Check sheet for the modelled part. Datum: model origin and axes. Units: mm. Give positions to 0.01 mm unless a question says otherwise; leave off trailing zeros. Order: outer loops, then holes, each group sorted by start corner. A loop starts at its lowest first (then second) coordinate and runs counter-clockwise, first axis right, second up.
Item 1: Material ranges on line 1 along X through (y, z) = (40, 1.9); line 2 along Y through (x, z) = (-79.5, 2.5); line 3 along X through (y, z) = (-140, 2.8), recorded low to high.
Item 2: Sectioned sample at C-C on z = 2. Count the separate pieces of the cut face and the enclosed holes in it, and give its area (3 significant figures).
Item 3: Sectioned sample at A-A on x = 3. Record the boundary of the cut face in (y, z) (3 decimals), and give its area (3 significant figures).
Item 4: Sectioned sample at B-B on x = 147. Record the boundary of the cut face in (y, z) (3 decimals).
from build123d import *

# Parameters (mm, degrees)
F0_R     = 1.984375
F0_W     = 38.1
F0_H     = 3.302
F0_W_2   = 3.302
F0_H_2   = 50.8
F0_W_3   = 79.248
F0_H_3   = 275.232702
F0_W_4   = 152.4
F0_H_4   = 254
F1_DEPTH = 3.175


with BuildPart() as f1:
    # F0 (on Top) → F1 (new body)
    with BuildSketch(Plane.XY):
        Polygon((-107.700216, 150.306364), (-206.125216, 150.306364), (-206.125216, -167.193636), (-107.700216, -167.193636), (114.549784, -167.193636), (212.974784, -167.193636), (212.974784, 150.306364), (114.549784, 150.306364), align=None)
        with Locations((-199.775216, -110.043636)):
            Circle(F0_R, mode=Mode.SUBTRACT)
        with Locations((-199.775216, -97.343636)):
            Circle(F0_R, mode=Mode.SUBTRACT)
        with Locations((-85.475216, -151.191636)):
            Circle(F0_R, mode=Mode.SUBTRACT)
        with Locations((-66.171216, -159.192636)):
            Rectangle(F0_W, F0_H, mode=Mode.SUBTRACT)
        with Locations((-72.775216, -151.191636)):
            Circle(F0_R, mode=Mode.SUBTRACT)
        with Locations((-60.075216, -151.191636)):
            Circle(F0_R, mode=Mode.SUBTRACT)
        with Locations((-47.375216, -151.191636)):
            Circle(F0_R, mode=Mode.SUBTRACT)
        with Locations((-34.675216, -151.191636)):
            Circle(F0_R, mode=Mode.SUBTRACT)
        with Locations((3.424784, -159.192636)):
            Rectangle(F0_W, F0_H, mode=Mode.SUBTRACT)
        with Locations((-199.775216, -84.643636)):
            Circle(F0_R, mode=Mode.SUBTRACT)
        with Locations((-191.774216, -84.643636)):
            Rectangle(F0_W_2, F0_H_2, mode=Mode.SUBTRACT)
        with Locations((-199.775216, -71.943636)):
            Circle(F0_R, mode=Mode.SUBTRACT)
        with Locations((-199.775216, -59.243636)):
            Circle(F0_R, mode=Mode.SUBTRACT)
        with Locations((-102.874216, -84.643636)):
            Rectangle(F0_W_2, F0_H_2, mode=Mode.SUBTRACT)
        with Locations((-86.872216, -84.643636)):
            Rectangle(F0_W_2, F0_H_2, mode=Mode.SUBTRACT)
        with Locations((41.524784, -151.191636)):
            Circle(F0_R, mode=Mode.SUBTRACT)
        with Locations((54.224784, -151.191636)):
            Circle(F0_R, mode=Mode.SUBTRACT)
        with Locations((73.020784, -159.192636)):
            Rectangle(F0_W, F0_H, mode=Mode.SUBTRACT)
        with Locations((66.924784, -151.191636)):
            Circle(F0_R, mode=Mode.SUBTRACT)
        with Locations((79.624784, -151.191636)):
            Circle(F0_R, mode=Mode.SUBTRACT)
        with Locations((92.324784, -151.191636)):
            Circle(F0_R, mode=Mode.SUBTRACT)
        with Locations((206.624784, -110.043636)):
            Circle(F0_R, mode=Mode.SUBTRACT)
        with Locations((206.624784, -97.343636)):
            Circle(F0_R, mode=Mode.SUBTRACT)
        with Locations((93.721784, -84.643636)):
            Rectangle(F0_W_2, F0_H_2, mode=Mode.SUBTRACT)
        with Locations((109.723784, -84.643636)):
            Rectangle(F0_W_2, F0_H_2, mode=Mode.SUBTRACT)
        with Locations((198.623784, -84.643636)):
            Rectangle(F0_W_2, F0_H_2, mode=Mode.SUBTRACT)
        with Locations((206.624784, -84.643636)):
            Circle(F0_R, mode=Mode.SUBTRACT)
        with Locations((206.624784, -71.943636)):
            Circle(F0_R, mode=Mode.SUBTRACT)
        with Locations((206.624784, -59.243636)):
            Circle(F0_R, mode=Mode.SUBTRACT)
        with Locations((-191.774216, -8.443636)):
            Rectangle(F0_W_2, F0_H_2, mode=Mode.SUBTRACT)
        with Locations((-147.324216, -5.242554)):
            Rectangle(F0_W_3, F0_H_3, mode=Mode.SUBTRACT)
        with Locations((-102.874216, -8.443636)):
            Rectangle(F0_W_2, F0_H_2, mode=Mode.SUBTRACT)
        with Locations((-199.775216, 42.356364)):
            Circle(F0_R, mode=Mode.SUBTRACT)
        with Locations((-199.775216, 55.056364)):
            Circle(F0_R, mode=Mode.SUBTRACT)
        with Locations((-199.775216, 67.756364)):
            Circle(F0_R, mode=Mode.SUBTRACT)
        with Locations((-191.774216, 67.756364)):
            Rectangle(F0_W_2, F0_H_2, mode=Mode.SUBTRACT)
        with Locations((-102.874216, 67.756364)):
            Rectangle(F0_W_2, F0_H_2, mode=Mode.SUBTRACT)
        with Locations((-86.872216, -8.443636)):
            Rectangle(F0_W_2, F0_H_2, mode=Mode.SUBTRACT)
        with Locations((3.424784, -8.443636)):
            Rectangle(F0_W_4, F0_H_4, mode=Mode.SUBTRACT)
        with Locations((-86.872216, 67.756364)):
            Rectangle(F0_W_2, F0_H_2, mode=Mode.SUBTRACT)
        with Locations((-199.775216, 80.456364)):
            Circle(F0_R, mode=Mode.SUBTRACT)
        with Locations((-199.775216, 93.156364)):
            Circle(F0_R, mode=Mode.SUBTRACT)
        with Locations((-85.475216, 134.304364)):
            Circle(F0_R, mode=Mode.SUBTRACT)
        with Locations((-72.775216, 134.304364)):
            Circle(F0_R, mode=Mode.SUBTRACT)
        with Locations((-60.075216, 134.304364)):
            Circle(F0_R, mode=Mode.SUBTRACT)
        with Locations((-66.171216, 142.305364)):
            Rectangle(F0_W, F0_H, mode=Mode.SUBTRACT)
        with Locations((-47.375216, 134.304364)):
            Circle(F0_R, mode=Mode.SUBTRACT)
        with Locations((-34.675216, 134.304364)):
            Circle(F0_R, mode=Mode.SUBTRACT)
        with Locations((3.424784, 142.305364)):
            Rectangle(F0_W, F0_H, mode=Mode.SUBTRACT)
        with Locations((93.721784, -8.443636)):
            Rectangle(F0_W_2, F0_H_2, mode=Mode.SUBTRACT)
        with Locations((93.721784, 67.756364)):
            Rectangle(F0_W_2, F0_H_2, mode=Mode.SUBTRACT)
        with Locations((109.723784, -8.443636)):
            Rectangle(F0_W_2, F0_H_2, mode=Mode.SUBTRACT)
        with Locations((154.173784, -5.242554)):
            Rectangle(F0_W_3, F0_H_3, mode=Mode.SUBTRACT)
        with Locations((198.623784, -8.443636)):
            Rectangle(F0_W_2, F0_H_2, mode=Mode.SUBTRACT)
        with Locations((109.723784, 67.756364)):
            Rectangle(F0_W_2, F0_H_2, mode=Mode.SUBTRACT)
        with Locations((206.624784, 42.356364)):
            Circle(F0_R, mode=Mode.SUBTRACT)
        with Locations((206.624784, 55.056364)):
            Circle(F0_R, mode=Mode.SUBTRACT)
        with Locations((198.623784, 67.756364)):
            Rectangle(F0_W_2, F0_H_2, mode=Mode.SUBTRACT)
        with Locations((206.624784, 67.756364)):
            Circle(F0_R, mode=Mode.SUBTRACT)
        with Locations((41.524784, 134.304364)):
            Circle(F0_R, mode=Mode.SUBTRACT)
        with Locations((54.224784, 134.304364)):
            Circle(F0_R, mode=Mode.SUBTRACT)
        with Locations((66.924784, 134.304364)):
            Circle(F0_R, mode=Mode.SUBTRACT)
        with Locations((79.624784, 134.304364)):
            Circle(F0_R, mode=Mode.SUBTRACT)
        with Locations((73.020784, 142.305364)):
            Rectangle(F0_W, F0_H, mode=Mode.SUBTRACT)
        with Locations((92.324784, 134.304364)):
            Circle(F0_R, mode=Mode.SUBTRACT)
        with Locations((206.624784, 80.456364)):
            Circle(F0_R, mode=Mode.SUBTRACT)
        with Locations((206.624784, 93.156364)):
            Circle(F0_R, mode=Mode.SUBTRACT)
    extrude(amount=F1_DEPTH)


solid = f1.part
Report:
1. line 1: x = -206.13 to -186.95, -107.7 to -72.78, 79.62 to 114.55, 193.8 to 212.97
1. line 2: y = -167.19 to -160.84, -157.54 to 140.65, 143.96 to 150.31
1. line 3: x = -206.13 to -186.95, -107.7 to 114.55, 193.8 to 212.97
2. separate pieces: 1
2. enclosed holes: 67
2. area: 46,500 mm2
3. outline: (-167.194, 0) - (-160.844, 0) - (-160.844, 3.175) - (-167.194, 3.175) - close; (-157.542, 0) - (-135.444, 0) - (-135.444, 3.175) - (-157.542, 3.175) - close; (118.556, 0) - (140.654, 0) - (140.654, 3.175) - (118.556, 3.175) - close; (143.956, 0) - (150.306, 0) - (150.306, 3.175) - (143.956, 3.175) - close
3. area: 181 mm2
4. outline: (-167.194, 0) - (-142.859, 0) - (-142.859, 3.175) - (-167.194, 3.175) - close; (132.374, 0) - (150.306, 0) - (150.306, 3.175) - (132.374, 3.175) - close
